The listing builds one solid part. Answer for the finished solid, in the listing's coordinates (mm). A direction names the side the tool comes from. Give positions to 0.01 mm unless a question says otherwise; leave off trailing zeros. Write each loop counter-clockwise with the first axis right and the second up, starting at its lowest first coordinate (ties: lowest second). Pieces come first, ordered by that corner, then holes. Notation, with made-up numbers: (77, 71.25) - (94, 71.25) arc R27 cw to (94, 98.25) - close; hole circle Ø9 at (63, 66.5). An arc over 180 degrees is marked (long way). Return JSON: item names as keys, results as strings.
from build123d import *

# Parameters (mm, degrees)
F1_DEPTH     = 10.25
F3_DEPTH     = 2.5
F5_T         = 1.9
F5_T3_DEPTH  = 32.8875665362
F5_T5_DEPTH  = 6.3
F5_T8_ANGLE  = 90.000000001
F5_T10_ANGLE = 90.000000001


# Not quite as in the source:
# - a shell that OpenCascade refuses in one call is made with other operations: the cavity is built on its own and cut out


with BuildPart() as f1:
    # F0 (on Top) → F1 (new body)
    with BuildSketch(Plane.XY):
        with BuildLine():
            Line((14, 19), (-18, 19))
            ThreePointArc((-18, 19), (-23.6568542495, 16.6568542495), (-26, 11))
            Line((-26, 11), (-26, -11))
            ThreePointArc((-26, -11), (-23.6568542495, -16.6568542495), (-18, -19))
            Line((-18, -19), (14, -19))
            ThreePointArc((14, -19), (19.6568542495, -16.6568542495), (22, -11))
            Line((22, -11), (22, 11))
            ThreePointArc((22, 11), (19.6568542495, 16.6568542495), (14, 19))
        make_face()
    extrude(amount=F1_DEPTH)

    # F2 (on face) → F3 (join)
    with BuildSketch(Plane.XY.offset(10.25)):
        with BuildLine():
            Line((11.0875665362, 21.85), (-18, 21.85))
            ThreePointArc((-18, 21.85), (-23.6568542495, 19.5068542495), (-26, 13.85))
            Line((-26, 13.85), (-26, -13.85))
            ThreePointArc((-26, -13.85), (-23.6568542495, -19.5068542495), (-18, -21.85))
            Line((-18, -21.85), (11.0875665362, -21.85))
            Line((11.0875665362, -21.85), (11.0875665362, 21.85))
        make_face()
    extrude(amount=-F3_DEPTH)

    # F5: shell of thickness 1.9, made by hand


with BuildPart() as f5_core1:
    # F5_t2: copy of F1
    add(f1.part)

    # the walls: a layer under each face that stays
    f5_faces = [f5_core1.faces().sort_by_distance(p)[0] for p in [
        (-2, 19, 5.125),
        (19.6568542495, 16.6568542495, 5.125),
        (22, 0, 5.125),
        (19.6568542495, -16.6568542495, 5.125),
        (-2, -19, 5.125),
        (-23.6568542495, -16.6568542495, 3.875),
        (-26, 0, 5.125),
        (-23.6568542495, -19.5068542495, 9),
        (-3.4562167319, -21.85, 9),
        (-23.6568542495, 19.5068542495, 9),
        (-3.4562167319, 21.85, 9),
        (-19.8187389106, -20.0416666667, 7.75),
        (11.0875665362, -20.425, 9),
        (-2, 0, 10.25),
        (11.0875665362, 20.425, 9),
        (-19.8187389106, 20.0416666667, 7.75),
        (-23.6568542495, 16.6568542495, 3.875),
    ]]
    thicken(f5_faces, amount=-F5_T, mode=Mode.SUBTRACT)

    # F5_s4 → F5_t3 (cut)
    with BuildSketch(Plane.YZ.offset(-19.9)):
        Polygon((19.019, 7.731), (17.1, 7.75), (17.1, 9.65), (19, 9.65), align=None)
        Polygon((-19.019, 7.731), (-17.1, 7.75), (-17.1, 9.65), (-19, 9.65), align=None)
    extrude(amount=F5_T3_DEPTH, mode=Mode.SUBTRACT)

    # F5_s6 → F5_t5 (cut)
    with BuildSketch(Plane.XY.offset(5.85)):
        Polygon((11.1065665362, 19.019), (11.0875665362, 17.1), (9.1875665362, 17.1), (9.1875665362, 19), align=None)
        Polygon((11.1065665362, -19.019), (11.0875665362, -17.1), (9.1875665362, -17.1), (9.1875665362, -19), align=None)
    extrude(amount=F5_T5_DEPTH, mode=Mode.SUBTRACT)

    # F5_s7 → F5_t8 (revolve, cut)
    with BuildSketch(Plane.YZ.offset(-18)):
        Polygon((-19.019, 7.731), (-17.1, 7.75), (-17.1, 9.65), (-19, 9.65), align=None)
    revolve(axis=Axis((-18, -11, 7.75), (0, 0, -1)), revolution_arc=F5_T8_ANGLE, mode=Mode.SUBTRACT)

    # F5_s9 → F5_t10 (revolve, cut)
    with BuildSketch(Plane.XZ.offset(-11)):
        Polygon((-26.019, 7.731), (-26, 9.65), (-24.1, 9.65), (-24.1, 7.75), align=None)
    revolve(axis=Axis((-18, 11, 7.75), (0, 0, -1)), revolution_arc=F5_T10_ANGLE, mode=Mode.SUBTRACT)


with BuildPart() as f1_1:
    add(f1.part)

    # what is left inside the walls is the cavity
    f5_cavity = [f5_core1.part.solids().sort_by_distance(p)[0] for p in [
        (-2, -5.7, 0.019),
    ]]
    add(f5_cavity, mode=Mode.SUBTRACT)


solid = f1_1.part
Item 1: A cutting plane is placed at C-C on y = 10. Determine the outline of the cut face in (x, z), then the cut area to 3 significant figures.
Answer below:
{"outline": "(-26, 0) - (-24.1, 0) - (-24.1, 8.35) - (20.1, 8.35) - (20.1, 0) - (22, 0) - (22, 10.25) - (-26, 10.25) - close", "area": "123 mm²"}
Item 2: The mould has two halves that part along Y. Classify faces 1 (the face through (-4, -21.85, 9)), 2 (the face through (-26, 0, 5)), 3 (the face through (18.266, -15.361, 4.117)), 4 (the face through (-2, 0, 8.35)): +Y half, -Y half, draft (parallel to the pull), parting line (faces both ways), or undercut.
Answer below:
{"face 1": "-Y half", "face 2": "draft", "face 3": "undercut", "face 4": "undercut"}
Item 3: A cutting plane is placed at A-A on z = 6.5. Determine the outline of the cut face in (x, y).
Answer below:
{"outline": "(-26, -11) arc R8 ccw to (-18, -19) - (14, -19) arc R8 ccw to (22, -11) - (22, 11) arc R8 ccw to (14, 19) - (-18, 19) arc R8 ccw to (-26, 11) - close; hole (-24.1, -11) arc R6.1 ccw to (-18, -17.1) - (14, -17.1) arc R6.1 ccw to (20.1, -11) - (20.1, 11) arc R6.1 ccw to (14, 17.1) - (-18, 17.1) arc R6.1 ccw to (-24.1, 11) - close"}
Item 4: For faces 5 (the face through (20.1, 0, 4)), 6 (the face through (-23.719, -16.594, 3.821)), 7 (the face through (-23.594, 16.719, 3.821)), determine the directions among +Z, -Z, +X, -X, +Y, -Y from which every point of the face is accessible in a straight line to the end or side of a thin tool.
Answer below:
{"face 5": "-Z", "face 6": "-Z, -X, -Y", "face 7": "-Z, -X, +Y"}
Item 5: A cutting plane is placed at B-B on x = 4. Determine the outline of the cut face in (y, z).
Answer below:
{"outline": "(-21.85, 7.75) - (-19, 7.75) - (-19, 0) - (-17.1, 0) - (-17.1, 8.35) - (17.1, 8.35) - (17.1, 0) - (19, 0) - (19, 7.75) - (21.85, 7.75) - (21.85, 10.25) - (-21.85, 10.25) - close"}
Item 6: A cutting plane is placed at D-D on x = 12. Determine the outline of the cut face in (y, z).
Answer below:
{"outline": "(-19, 0) - (-17.1, 0) - (-17.1, 8.35) - (17.1, 8.35) - (17.1, 0) - (19, 0) - (19, 10.25) - (-19, 10.25) - close"}
Item 7: Consider L1, parallel to X at y = -10.5, z = 2; L2, parallel to Y at x = -4, z = 8.25; L3, parallel to Y at x = -9, z = 1.75. Determine where each line is inside the solid, lowest interval first.
Answer below:
{"L1": "x = -26 to -24.1, 20.1 to 22", "L2": "y = -21.85 to -17.1, 17.1 to 21.85", "L3": "y = -19 to -17.1, 17.1 to 19"}
Item 8: Flat-ended cylindrical pins translate along their axes: P1, Ø5, axis at x = -9, z = 2.5, coming from the +Y side; P2, Ø0.8, axis at y = -20, z = 8.5, coming from the +X side; P3, Ø2.5, axis at x = -1, z = 3, coming from the -Y side. Find the tip coordinate at first contact, or state that the pin passes through.
Answer below:
{"P1": "stops at y = 19", "P2": "stops at x = 11.09", "P3": "stops at y = -19"}
